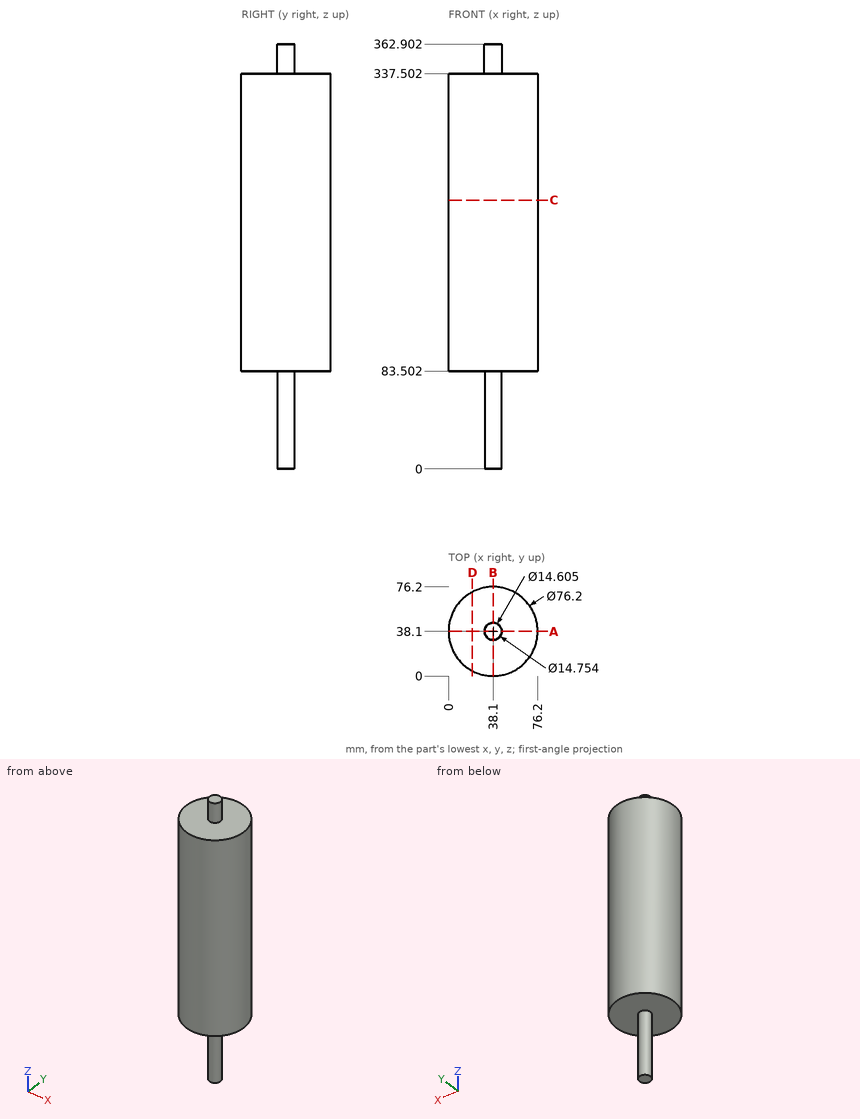
Could you check a few things on this drawing? It's one solid part, dimensions in mm from its lowest x, y, z. Round coordinates to 2 decimals unless told otherwise and drop trailing zeros. Loops run counter-clockwise (first coordinate to the right, second up) from the corner with the lowest first, then second, coordinate; pieces in that order, holes last. Notation, with made-up numbers: (15, -22.75) -> (45, -22.75) arc R12 cw to (45, -10.75) -> close; hole circle Ø6 at (33, -5). An arc over 180 degrees is marked (long way). One line per item, written item: value. Start each with the question number.
1. If we section it at D-D, the plane x = 20.5: Write out the boundary of the cut face in (y, z), then the cut area to 3 significant figures.
2. If we section it at A-A, the plane y = 38.1: Write out the boundary of the cut face in (x, z), then the cut area to 4 significant figures.
3. If we section it at C-C, the plane z = 229.5: Write out the boundary of the cut face in (x, y).
4. If I drill on probe 1 along Z at (x, y) = (43.5, 19.5); probe 2 along Y at (x, z) = (39, 246.5); probe 3 along Y at (x, z) = (72, 91.5) (1 decimal), over which ranges is the centre line in solid material (lowest first)?
5. For pin 1 (8 mm diameter, centred on x = 7.5, z = 280.5, fed in from -Y); pin 2 (8 mm diameter, centred on x = 52, y = 61.5, fed in from -Z); pin 3 (3 mm diameter, centred on y = 40, z = 245, fed in from +X), each with a flat end and sliding along its axis, tell me the tip position at first contact or that it passes through.
Calculated:
1. outline: (4.31, 83.5) -> (71.89, 83.5) -> (71.89, 337.5) -> (4.31, 337.5) -> close
1. area: 17,200 mm²
2. outline: (0, 83.5) -> (30.8, 83.5) -> (30.8, 0) -> (45.4, 0) -> (45.4, 83.5) -> (76.2, 83.5) -> (76.2, 337.5) -> (45.48, 337.5) -> (45.48, 362.9) -> (30.72, 362.9) -> (30.72, 337.5) -> (0, 337.5) -> close
2. area: 20,950 mm²
3. outline: circle Ø76.2 at (38.1, 38.1)
4. probe 1: z = 83.5 to 337.5
4. probe 2: y = 0.01 to 76.19
4. probe 3: y = 20.7 to 55.5
5. pin 1: stops at y = 10.82
5. pin 2: stops at z = 83.5
5. pin 3: stops at x = 76.2
